from build123d import *

# Parameters (mm, degrees)
F0_W     = 648
F0_H     = 50
F1_DEPTH = 6
F2_W     = 648
F2_H     = 6
F3_DEPTH = 44
F4_R     = 9
F5_DEPTH = 50.001


with BuildPart() as f1:
    # F0 (on Front) → F1 (new body)
    with BuildSketch(Plane.XZ):
        with Locations((324, 25)):
            Rectangle(F0_W, F0_H)
    extrude(amount=F1_DEPTH)

    # F2 (on face) → F3 (join)
    with BuildSketch(Plane(origin=(0, 0, 0), x_dir=(-1, 0, 0), z_dir=(0, 1, 0))):
        with Locations((-324, 47)):
            Rectangle(F2_W, F2_H)
    extrude(amount=F3_DEPTH)

    # F4 (on face) → F5 (cut, through all)
    with BuildSketch(Plane.XZ.offset(6)):
        with Locations((25, 22)):
            Circle(F4_R)
        with Locations((623, 22)):
            Circle(F4_R)
    extrude(amount=-F5_DEPTH, mode=Mode.SUBTRACT)


solid = f1.part
The listing builds one solid part. Answer for the finished solid, in the listing's coordinates (mm). A direction names the side the tool comes from. Give positions to 0.01 mm unless a question says otherwise; leave off trailing zeros. Write each loop counter-clockwise with the first axis right and the second up, starting at its lowest first coordinate (ties: lowest second). Pieces come first, ordered by that corner, then holes. Notation, with made-up numbers: (72.25, 71.25) - (102.25, 71.25) arc R20 ccw to (102.25, 80.25) - close; hole circle Ø9 at (-31.75, 2). An arc over 180 degrees is marked (long way). One line per question, with ' | ' between items. Start each with the question number.
1. Section B-B, the plane x = 623 is taken. Determine the outline of the cut face in (y, z).
2. For faces 4 (the face through (329, 19, 50)), 5 (the face through (319, 0, 22)), determine the directions among +Z, -Z, +X, -X, +Y, -Y from which every point of the face is accessible in a straight line to the end or side of a thin tool.
3. Determine the mould class of faces 1 (the face through (33.584, -3.042, 24.703)), 2 (the face through (0, -1, 34)), 3 (the face through (329, 22, 44)) for opening direction Z: +Z half, -Z half, draft (parallel to the pull), parting line (faces both ways), or undercut.
4. Section D-D, the plane x = 275 is taken. Determine the outline of the cut face in (y, z), then the cut area to 3 significant figures.
5. Given P1, Ø14.5, axis at x = 623, z = 22, coming from the -Y side; P2, Ø13, axis at x = 168, z = 11.5, coming from the +Y side; P3, Ø12, axis at x = 268, y = 17.5, coming from the -Z side, each flat-ended and moving along its own axis, determine where each tip first touches the part or whether it passes through.
6. Straight lines are drawn through the part: line 1 (Z direction, x = 623, y = -3.6); line 2 (Y direction, x = 534.5, z = 12.5); line 3 (Z direction, x = 247, y = 14). For each, find the intervals that lie inside material, in ascending order.
7. Section A-A, the plane z = 22 is taken. Determine the outline of the cut face in (x, y).
8. Section C-C, the plane y = 21 is taken. Determine the outline of the cut face in (x, z).
Result:
1) outline: (-6, 0) - (0, 0) - (0, 13) - (-6, 13) - close; (-6, 31) - (0, 31) - (0, 44) - (44, 44) - (44, 50) - (-6, 50) - close
2) face 4: +Z, +X, -X, +Y, -Y | face 5: -Z, +X, -X, +Y
3) face 1: undercut | face 2: draft | face 3: -Z half
4) outline: (-6, 0) - (0, 0) - (0, 44) - (44, 44) - (44, 50) - (-6, 50) - close | area: 564 mm2
5) P1: passes through | P2: stops at y = 0 | P3: stops at z = 44
6) line 1: z = 0 to 13, 31 to 50 | line 2: y = -6 to 0 | line 3: z = 44 to 50
7) outline: (0, -6) - (16, -6) - (16, 0) - (0, 0) - close; (34, -6) - (614, -6) - (614, 0) - (34, 0) - close; (632, -6) - (648, -6) - (648, 0) - (632, 0) - close
8) outline: (0, 44) - (648, 44) - (648, 50) - (0, 50) - close
